Read the model definition and answer for the solid it produces. Units are mm, in the model's axes. A direction names the side the tool comes from. Give positions to 0.01 mm unless a question says otherwise; leave off trailing zeros. Loops run counter-clockwise (first coordinate to the right, second up) from the corner with the lowest first, then second, coordinate; pieces in that order, holes last. Notation, with made-up numbers: (30.25, 18.25) - (38.25, 18.25) arc R13 ccw to (38.25, 24.25) - close; hole circle Ø2 at (85.25, 64). An arc over 180 degrees is marked (long way). Use a Markdown table: item, result. Add a question column.
Item 1: Each of these flat-tipped pins is pushed along its axis until it touches: P1, Ø5.5, axis at x = 1, y = -3, coming from the -Z side; P2, Ø2.5, axis at y = 8, z = 11.5, coming from the -X side; P3, Ø1.5, axis at x = -1, y = -5, coming from the +Z side. Where does it stop, or does it pass through?
Item 2: A cutting plane is placed at A-A (y = -3.5). Determine the outline of the cut face in (x, z).
Item 3: Consider probe 1 along Z at (x, y) = (-0.25, 4.25); probe 2 along X at (y, z) = (1.75, -10.25); probe 3 along Y at (x, z) = (4, 9). Determine where each line is inside the solid, lowest interval first. Write a range as [from, to].
Item 4: For a pull along Z with two mould halves and no side action, classify faces 5 (the face through (0, -4, 0.5)), 6 (the face through (0, -4, -0.5)), 7 (the face through (2, 6, -11)) as +Z half, -Z half, draft (parallel to the pull), parting line (faces both ways), or undercut.
Item 5: Which of the six approach directions +Z, -Z, +X, -X, +Y, -Y give full straight-line access (tool end or side, diameter ignored) to faces 1 (the face through (-2.5, -4, 0)), 2 (the face through (0, -4, -6.5)), 3 (the face through (0, 6, 12.5)), 4 (the face through (0, -4, -7.5))?
from build123d import *

# Parameters (mm, degrees)
BOSS_EXTRU_1_DEPTH = 13
BOSS_EXTRU_2_DEPTH = 2
CONG_1_R           = 2
ESQUISSE3_W        = 5
ESQUISSE3_H        = 1
BOSS_EXTRU_3_DEPTH = 9


# Read off the part's stored shape, not the designer's step: Boss.-Extru.2
with BuildPart() as part:
    # Esquisse1 → Boss.-Extru.1 (new body)
    with BuildSketch(Plane(origin=(0, 0, 0), x_dir=(1, 0, 0), z_dir=(0, 1, 0))):
        with BuildLine():
            Line((2, 10.062305899), (2, 12.5))
            Line((2, 12.5), (-2, 12.5))
            Line((-2, 12.5), (-2, 10.062305899))
            add(Edge.make_bspline(
                [(-2, 10.062305899), (-24.5, 0), (-2, -10.062305899)],
                knots=[3.431344355, 3.431344355, 3.431344355, 5.993433606, 5.993433606, 5.993433606], degree=2, weights=[1, 0.285714286, 1]))
            Line((-2, -10.062305899), (-2, -12.5))
            Line((-2, -12.5), (2, -12.5))
            Line((2, -12.5), (2, -10.062305899))
            add(Edge.make_bspline(
                [(2, -10.062305899), (24.5, 0), (2, 10.062305899)],
                knots=[0.289751701, 0.289751701, 0.289751701, 2.851840952, 2.851840952, 2.851840952], degree=2, weights=[1, 0.285714286, 1]))
        make_face()
    extrude(amount=BOSS_EXTRU_1_DEPTH)

    # Boss.-Extru.2 outline → Boss.-Extru.2 (add)
    with BuildSketch(Plane(origin=(0, 13, 0), x_dir=(1, 0, 0), z_dir=(0, 1, 0))):
        with BuildLine():
            add(Edge.make_bspline(
                [(0, -13), (0.703240737, -13), (2.109722211, -12.789689498), (4.688231544, -11.602625859), (7.229672734, -8.991447827), (9.080604982, -4.777577384), (9.709697509, 0), (9.080604982, 4.777577384), (7.229672734, 8.991447827), (4.688231544, 11.602625859), (2.109722211, 12.789689498), (0, 13.105155251), (-2.109722211, 12.789689498), (-4.688231544, 11.602625859), (-7.229672734, 8.991447827), (-9.080604982, 4.777577384), (-9.709697509, 0), (-9.080604982, -4.777577384), (-7.229672734, -8.991447827), (-4.688231544, -11.602625859), (-2.109722211, -12.789689498), (-0.703240737, -13), (0, -13)],
                knots=[0, 0, 0, 0, 0.196349541, 0.392699082, 0.785398163, 1.178097245, 1.570796327, 1.963495408, 2.35619449, 2.748893572, 2.945243113, 3.141592654, 3.337942194, 3.534291735, 3.926990817, 4.319689899, 4.71238898, 5.105088062, 5.497787144, 5.890486225, 6.086835766, 6.283185307, 6.283185307, 6.283185307, 6.283185307], degree=3))
        make_face()
    extrude(amount=BOSS_EXTRU_2_DEPTH)

    # Congé1
    cong_1_edges = [part.edges().sort_by_distance(p)[0] for p in [
        (0, 15, -13),
    ]]
    fillet(cong_1_edges, radius=CONG_1_R - 0.0004)  # a hair under: the kernel refuses the full size

    # Esquisse3 → Boss.-Extru.3 (add)
    with BuildSketch(Plane.XZ):
        Rectangle(ESQUISSE3_W, ESQUISSE3_H)
        with Locations((0, -7)):
            Rectangle(ESQUISSE3_W, ESQUISSE3_H)
    extrude(amount=BOSS_EXTRU_3_DEPTH)


solid = part.part
Geometry says:
| question | item | result |
|---|---|---|
| 1 | P1 | z = -7.5 |
| 1 | P2 | x = -2 |
| 1 | P3 | z = 0.5 |
| 2 | outline | (-2.5, -7.5) - (2.5, -7.5) - (2.5, -6.5) - (-2.5, -6.5) - close; (-2.5, -0.5) - (2.5, -0.5) - (2.5, 0.5) - (-2.5, 0.5) - close |
| 3 | probe 1 | [-12.5, 12.5] |
| 3 | probe 2 | [-2, 2] |
| 3 | probe 3 | [13, 15] |
| 4 | face 5 | +Z half |
| 4 | face 6 | undercut |
| 4 | face 7 | draft |
| 5 | face 1 | +Z, -Z, -X, -Y |
| 5 | face 2 | +X, -X, -Y |
| 5 | face 3 | +Z, +X, -X, -Y |
| 5 | face 4 | -Z, +X, -X, -Y |
